```python
from build123d import *

# Parameters (mm, degrees)
SKETCH2_R           = 13
SKETCH2_R_2         = 11
BOSS_EXTRUDE3_DEPTH = 98.5
CUT_EXTRUDE2_START  = 7
SKETCH2_2_R         = 13
SKETCH2_2_R_2       = 11
CUT_EXTRUDE2_DEPTH  = 84.5
SKETCH1_W           = 30
SKETCH1_H           = 98.5
SKETCH1_R           = 2
BOSS_EXTRUDE5_DEPTH = 4
SKETCH3_W           = 8.573743233
SKETCH3_H           = 7
SKETCH3_W_2         = 12.852513534
SKETCH3_W_3         = 30
BOSS_EXTRUDE8_DEPTH = 24
SKETCH4_W           = 30
SKETCH4_H           = 12
BOSS_EXTRUDE9_DEPTH = 84.5
SKETCH2_3_R         = 11
CUT_EXTRUDE3_DEPTH  = 360.900226616
CUT_EXTRUDE4_START  = 3
SKETCH1_6_R         = 2
CUT_EXTRUDE4_DEPTH  = 10
SKETCH1_7_R         = 2
CUT_EXTRUDE5_DEPTH  = 427.557716632


with BuildPart() as part:
    # Sketch2 → Boss-Extrude3 (new body)
    with BuildSketch(Plane.XZ.offset(150.75)):
        with Locations(Location((-330, 15.300585116, 0), (0, 0, 180))):
            Circle(SKETCH2_R)
        with Locations(Location((-330, 15.300585116, 0), (0, 0, 242.228070503))):
            Circle(SKETCH2_R_2, mode=Mode.SUBTRACT)
    extrude(amount=BOSS_EXTRUDE3_DEPTH)

    # Sketch2<2> → Cut-Extrude2 (cut)
    with BuildSketch(Plane.XZ.offset(150.75).offset(CUT_EXTRUDE2_START)):
        with Locations((-330, 15.300585116)):
            Circle(SKETCH2_2_R)
        with Locations((-330, 15.300585116)):
            Circle(SKETCH2_2_R_2, mode=Mode.SUBTRACT)
    extrude(amount=CUT_EXTRUDE2_DEPTH, mode=Mode.SUBTRACT)


with BuildPart() as cut_extrude2_piece_1:
    # of the separate pieces the step leaves, piece 1, a body of its own (cut_extrude2_pieces)
    add(part.part.solids().sort_by_distance((-343, -150.75, 15.300585116))[0])

    # Sketch1 → Boss-Extrude5 (add)
    # profile 1 of 3: a face of its own
    with BuildSketch(Plane.XY):
        with Locations((-330, -200)):
            Rectangle(SKETCH1_W, SKETCH1_H)
        Polygon((-331.991858429, -235.55), (-333.983716857, -239), (-331.991858429, -242.45), (-328.008141571, -242.45), (-326.016283143, -239), (-328.008141571, -235.55), align=None, mode=Mode.SUBTRACT)
        Polygon((-328.008141571, -164.45), (-326.016283143, -161), (-328.008141571, -157.55), (-331.991858429, -157.55), (-333.983716857, -161), (-331.991858429, -164.45), align=None, mode=Mode.SUBTRACT)
    # profile 2 of 3: a face of its own
    with BuildSketch(Plane.XY):
        Polygon((-331.991858429, -164.45), (-328.008141571, -164.45), (-326.016283143, -161), (-328.008141571, -157.55), (-331.991858429, -157.55), (-333.983716857, -161), align=None)
        with Locations((-330, -161)):
            Circle(SKETCH1_R, mode=Mode.SUBTRACT)
    # profile 3 of 3: a face of its own
    with BuildSketch(Plane.XY):
        Polygon((-328.008141571, -235.55), (-331.991858429, -235.55), (-333.983716857, -239), (-331.991858429, -242.45), (-328.008141571, -242.45), (-326.016283143, -239), align=None)
        with Locations((-330, -239)):
            Circle(SKETCH1_R, mode=Mode.SUBTRACT)
    extrude(amount=BOSS_EXTRUDE5_DEPTH)



with BuildPart() as cut_extrude2_piece_2:
    # of the separate pieces the step leaves, piece 2, a body of its own (cut_extrude2_pieces)
    add(part.part.solids().sort_by_distance((-343, -242.25, 15.300585116))[0])


with BuildPart() as cut_extrude2_piece_1_1:
    add(cut_extrude2_piece_1.part)

    add(cut_extrude2_piece_2.part)  # Boss-Extrude8 merges Cut-Extrude2 piece 2
    # Sketch3 → Boss-Extrude8 (add)
    with BuildSketch(Plane.XY.offset(4)):
        with Locations((-340.713128384, -154.25)):
            Rectangle(SKETCH3_W, SKETCH3_H)
        with Locations((-330, -154.25)):
            Rectangle(SKETCH3_W_2, SKETCH3_H)
        with Locations((-330, -245.75)):
            Rectangle(SKETCH3_W_3, SKETCH3_H)
        with Locations((-319.286871616, -154.25)):
            Rectangle(SKETCH3_W, SKETCH3_H)
    extrude(amount=BOSS_EXTRUDE8_DEPTH)

    # Sketch4 → Boss-Extrude9 (add)
    with BuildSketch(Plane.XZ.offset(157.75)):
        with Locations((-330, 10)):
            Rectangle(SKETCH4_W, SKETCH4_H)
    extrude(amount=BOSS_EXTRUDE9_DEPTH)

    # Sketch2<3> → Cut-Extrude3 (cut, through all)
    with BuildSketch(Plane.XZ.offset(150.75)):
        with Locations((-330, 15.300585116)):
            Circle(SKETCH2_3_R)
    extrude(amount=CUT_EXTRUDE3_DEPTH, mode=Mode.SUBTRACT)

    # Sketch1<6> → Cut-Extrude4 (cut)
    # profile 1 of 2: a face of its own
    with BuildSketch(Plane.XY.offset(CUT_EXTRUDE4_START)):
        Polygon((-331.991858429, -164.45), (-328.008141571, -164.45), (-326.016283143, -161), (-328.008141571, -157.55), (-331.991858429, -157.55), (-333.983716857, -161), align=None)
        with Locations((-330, -161)):
            Circle(SKETCH1_6_R, mode=Mode.SUBTRACT)
    # profile 2 of 2: a face of its own
    with BuildSketch(Plane.XY.offset(CUT_EXTRUDE4_START)):
        Polygon((-328.008141571, -235.55), (-331.991858429, -235.55), (-333.983716857, -239), (-331.991858429, -242.45), (-328.008141571, -242.45), (-326.016283143, -239), align=None)
        with Locations((-330, -239)):
            Circle(SKETCH1_6_R, mode=Mode.SUBTRACT)
    extrude(amount=CUT_EXTRUDE4_DEPTH, mode=Mode.SUBTRACT)


with BuildPart() as cut_extrude4_piece_1:
    # of the separate pieces the step leaves, piece 1, a body of its own (cut_extrude4_pieces)
    add(cut_extrude2_piece_1_1.part.solids().sort_by_distance((-315, -249.25, 28))[0])


with BuildPart() as cut_extrude4_piece_2:
    # of the separate pieces the step leaves, piece 2, a body of its own (cut_extrude4_pieces)
    add(cut_extrude2_piece_1_1.part.solids().sort_by_distance((-328, -161, 4.48393129))[0])


with BuildPart() as cut_extrude4_piece_3:
    # of the separate pieces the step leaves, piece 3, a body of its own (cut_extrude4_pieces)
    add(cut_extrude2_piece_1_1.part.solids().sort_by_distance((-328, -239, 4.48393129))[0])


with BuildPart() as cut_extrude5_tool:
    # Sketch1<7> → Cut-Extrude5 (new, through all)
    with BuildSketch(Plane.XY):
        with Locations((-330, -161)):
            Circle(SKETCH1_7_R)
        with Locations((-330, -239)):
            Circle(SKETCH1_7_R)
    extrude(amount=CUT_EXTRUDE5_DEPTH)


with BuildPart() as cut_extrude4_piece_2_1:
    add(cut_extrude4_piece_2.part)

    # Cut-Extrude5: cut by cut_extrude5_tool
    add(cut_extrude5_tool.part, mode=Mode.SUBTRACT)


with BuildPart() as cut_extrude4_piece_3_1:
    add(cut_extrude4_piece_3.part)

    # Cut-Extrude5: cut by cut_extrude5_tool
    add(cut_extrude5_tool.part, mode=Mode.SUBTRACT)


solid = cut_extrude4_piece_1.part
```
Work out the finished part from the listing and answer in its coordinate system (mm). A direction names the side the tool comes from. Coordinates: 2 decimals unless noted, no trailing zeros. Order: outer loops, then holes, each group sorted by start corner. A loop starts at its lowest first (then second) coordinate and runs counter-clockwise, first axis right, second up. Notation, with made-up numbers: (33, -10) - (51, -10) arc R18 cw to (51, -6) - close; hole circle Ø6 at (-1, -31.75). An arc over 180 degrees is marked (long way). Answer as a JSON object with one key per item and string values.
1. Find section A-A on x = -330. Determine the outline of the cut face in (y, z).
Output values:
{"outline": "(-249.25, 0) - (-241, 0) - (-241, 3) - (-242.45, 3) - (-242.45, 4.3) - (-249.25, 4.3) - close; (-249.25, 26.3) - (-242.25, 26.3) - (-242.25, 28.3) - (-249.25, 28.3) - close; (-237, 0) - (-163, 0) - (-163, 3) - (-164.45, 3) - (-164.45, 4.3) - (-235.55, 4.3) - (-235.55, 3) - (-237, 3) - close; (-159, 0) - (-150.75, 0) - (-150.75, 4.3) - (-157.55, 4.3) - (-157.55, 3) - (-159, 3) - close; (-157.75, 26.3) - (-150.75, 26.3) - (-150.75, 28.3) - (-157.75, 28.3) - close"}
2. Find section B-B on z = 21.25. Determine the outline of the cut face in (x, y), plus the area to 3 significant figures.
Output values:
{"outline": "(-345, -249.25) - (-339.25, -249.25) - (-339.25, -242.25) - (-345, -242.25) - close; (-345, -157.75) - (-339.25, -157.75) - (-339.25, -150.75) - (-345, -150.75) - close; (-320.75, -249.25) - (-315, -249.25) - (-315, -242.25) - (-320.75, -242.25) - close; (-320.75, -157.75) - (-315, -157.75) - (-315, -150.75) - (-320.75, -150.75) - close", "area": "161 mm²"}
3. Consider line 1 (Y direction, x = -330, z = 1.6); line 2 (Y direction, x = -341.5, z = 25.75); line 3 (Z direction, x = -317, y = -160). Determine where each line is inside the solid, lowest interval first.
Output values:
{"line 1": "y = -249.25 to -241, -237 to -163, -159 to -150.75", "line 2": "y = -249.25 to -242.25, -157.75 to -150.75", "line 3": "z = 0 to 16"}
4. Find section C-C on y = -212. Determine the outline of the cut face in (x, z), plus the area to 3 significant figures.
Output values:
{"outline": "(-345, 0) - (-315, 0) - (-315, 16) - (-319.02, 16) arc R11 cw (long way) to (-340.98, 16) - (-345, 16) - close", "area": "275 mm²"}
5. A tool of negligible diameter and unlimited length cuts with its end or side. For faces 5 (the face through (-339, -154, 28)), 6 (the face through (-317, -199, 16)), 7 (the face through (-333, -162.7, 3.8)), 8 (the face through (-321, -246, 28)), from which of +Z, -Z, +X, -X, +Y, -Y can it reach the whole face along a straight path? Write none if from no direction.
Output values:
{"face 5": "+Z, -X, +Y, -Y", "face 6": "+Z, +X, -X", "face 7": "+Z", "face 8": "+Z, +X, +Y, -Y"}
6. Each of these flat-tipped pins is pushed along its axis until it touches: P1, Ø1, axis at x = -338.5, z = 12, coming from the +Y side; P2, Ø7.5, axis at x = -319, y = -246, coming from the +Z side; P3, Ø3.5, axis at x = -331.5, y = -160, coming from the +Z side; P4, Ø4.5, axis at x = -316.5, y = -202, coming from the +Z side. Where does it stop, or does it pass through?
Output values:
{"P1": "passes through", "P2": "stops at z = 28", "P3": "stops at z = 4.78", "P4": "stops at z = 16"}
7. The mould has two halves that part along Y. Classify faces 1 (the face through (-333, -159.3, 3.8)), 2 (the face through (-333, -237.3, 3.8)), 3 (the face through (-339, -246, 28)), 4 (the face through (-326.5, -249.25, 4.5)): +Y half, -Y half, draft (parallel to the pull), parting line (faces both ways), or undercut.
Output values:
{"face 1": "undercut", "face 2": "undercut", "face 3": "draft", "face 4": "-Y half"}
8. Find section D-D on z = 11.5. Determine the outline of the cut face in (x, y).
Output values:
{"outline": "(-345, -249.25) - (-340.32, -249.25) - (-340.32, -150.75) - (-345, -150.75) - close; (-319.68, -249.25) - (-315, -249.25) - (-315, -150.75) - (-319.68, -150.75) - close"}
